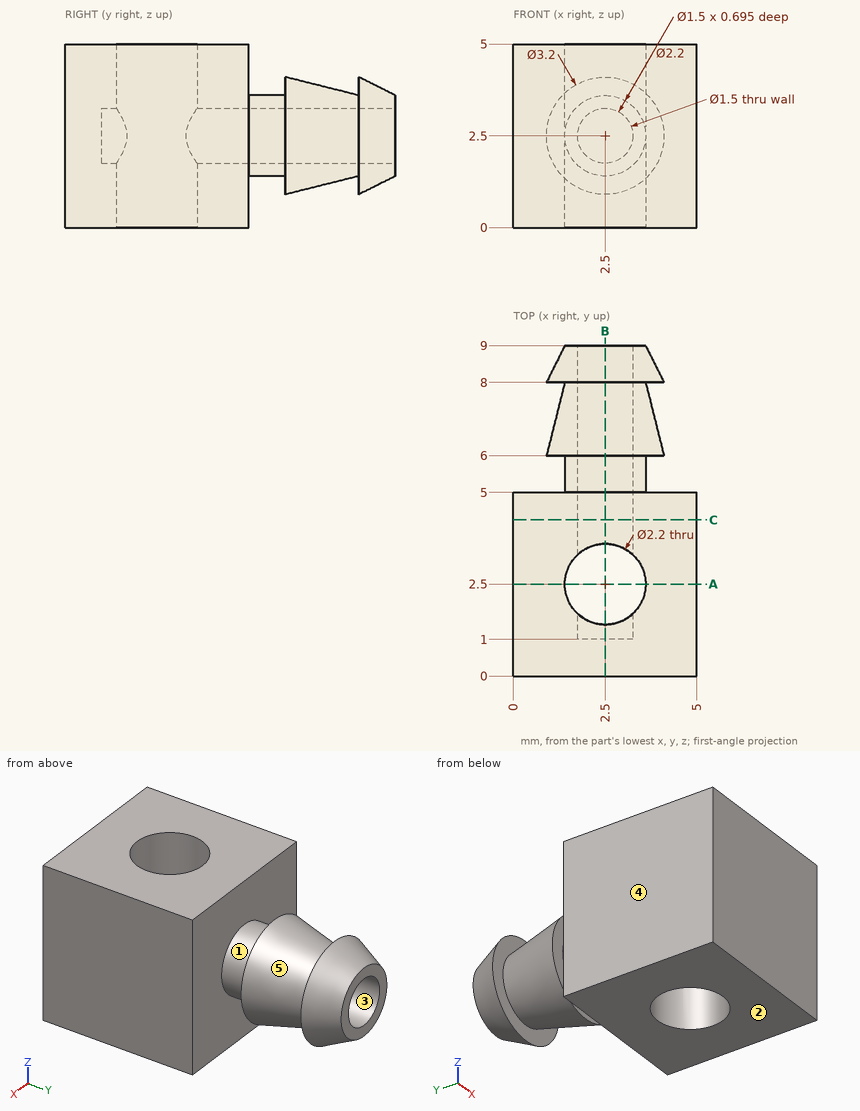
Job drawing, mm, ordinate dimensions from the low corner. One solid piece. A direction names the side the tool comes from. Round coordinates to 2 decimals unless told otherwise and drop trailing zeros. Order: outer loops, then holes, each group sorted by start corner. A loop starts at its lowest first (then second) coordinate and runs counter-clockwise, first axis right, second up. Notation, with made-up numbers: M 12.25,-22.75 L 54.25,-22.75 A10 cw 54.25,-7.75 Z; hole C 31,-10.75 d3. An arc over 180 degrees is marked long. Write each question's results on one line, items separated by ' | '. Start each with the question number.
(1) Which spindle directions (+Z, -Z, +X, -X, +Y, -Y) get a long thin tool onto all of the face, cutting with end or side? Do the marked faces 1 and 2. Say none if no direction does.
(2) Probe probe 1 along Y at (x, z) = (4.05, 4.3); probe 2 along Y at (x, z) = (2.4, 4.7) (1 decimal); probe 3 along X at (y, z) = (3, 0.8). List the from-to ranges inside material, lowest first. Write a range as from..to.
(3) Two-plate mould, pull along Z, no slides. Class the marked faces 3, 4 and 5: pulls with the +Z half, pulls with the -Z half, needs draft (parallel to the pull), parting line crosses it, or undercut.
(4) Saw through at C-C, the plane y = 4.25. Give the cut face in (x, z), then the cut area to 3 significant figures.
(5) Drop flat-ended pins along their axis: pin 1 (2 mm diameter, centred on x = 4, z = 3, fed in from -Y); pin 2 (0.8 mm diameter, centred on x = 2.5, z = 2.5, fed in from +Y); pin 3 (1.3 mm diameter, centred on x = 2.5, y = 2.5, fed in from -Z). Give the stop position or say it passes through.
(6) Saw through at A-A, the plane y = 2.5. Give the cut face in (x, z).
(7) Saw through at B-B, the plane x = 2.5. Give the cut face in (y, z), then the cut area to 3 significant figures.
Established:
1) face 1: none | face 2: -Z, +X, -X, +Y, -Y
2) probe 1: y = 0..5 | probe 2: y = 0..1.4, 3.6..5 | probe 3: x = 0..1.52, 3.48..5
3) face 3: undercut | face 4: needs draft | face 5: parting line crosses it
4) outline: M 0,0 L 5,0 L 5,5 L 0,5 Z; hole C 2.5,2.5 d1.5 | area: 23.2 mm^2
5) pin 1: stops at y = 0 | pin 2: stops at y = 1 | pin 3: passes through
6) outline: M 0,0 L 1.4,0 L 1.4,5 L 0,5 Z; M 3.6,0 L 5,0 L 5,5 L 3.6,5 Z
7) outline: M 0,0 L 1.4,0 L 1.4,1.75 L 1,1.75 L 1,3.25 L 1.4,3.25 L 1.4,5 L 0,5 Z; M 3.6,0 L 5,0 L 5,1.4 L 6,1.4 L 6,0.9 L 8,1.4 L 8,0.9 L 9,1.4 L 9,1.75 L 3.6,1.75 Z; M 3.6,3.25 L 9,3.25 L 9,3.6 L 8,4.1 L 8,3.6 L 6,4.1 L 6,3.6 L 5,3.6 L 5,5 L 3.6,5 Z | area: 15.6 mm^2
